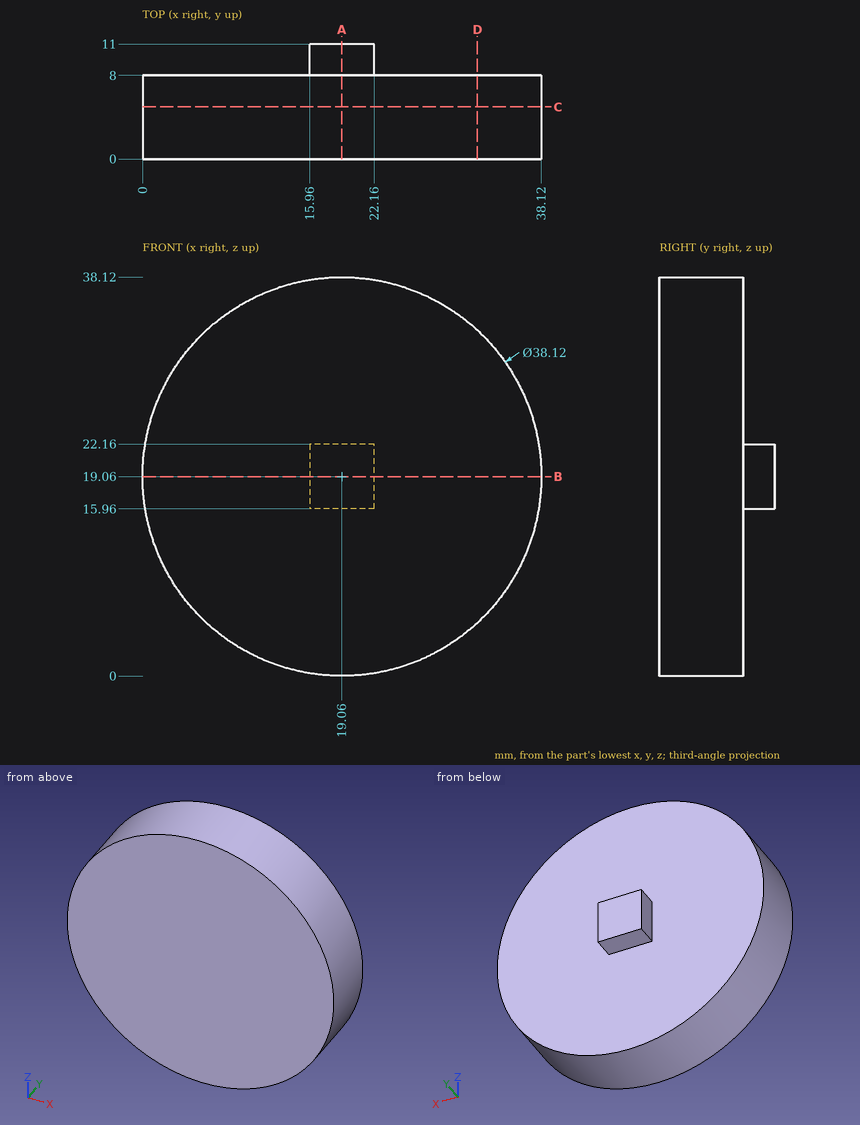
The figure shows three views and two pictorial views of one solid part (mm, origin at its lowest corner). Answer the questions. Round coordinates to 2 decimals unless told otherwise and drop trailing zeros. Order: outer loops, then holes, each group sorted by start corner. A loop starts at its lowest first (then second) coordinate and runs counter-clockwise, first axis right, second up. Notation, with made-up numbers: M -9.5,-18 L 40.5,-18 A18 ccw 40.5,13 Z; hole C 36,74.25 d9. An arc over 180 degrees is marked long. Put each result on its own line as item: value. Start each with the question number.
Q1. Section C-C, the plane y = 5 is taken. Write down the section's boundary in (x, z).
Q2. Straight lines are drawn through the part: L1, parallel to Y at x = 9, z = 33.5; L2, parallel to Z at x = 20, y = 10.25; L3, parallel to X at y = 5.75, z = 18.5. For each, find the intervals that lie inside material, in ascending order. Write a range as [from, to].
Q3. Flat-ended cylindrical pins translate along their axes: pin 1 (0.9 mm diameter, centred on x = 19, y = 9, fed in from -Z); pin 2 (1.5 mm diameter, centred on y = 10, z = 18, fed in from -X); pin 3 (2.5 mm diameter, centred on y = 9, z = 18, fed in from +X). Find the tip coordinate at first contact, or state that the pin passes through.
Q4. Section A-A, the plane x = 19.06 is taken. Write down the section's boundary in (y, z).
Q5. Section D-D, the plane x = 32 is taken. Write down the section's boundary in (y, z), and give its area (3 significant figures).
Q6. Section B-B, the plane z = 19.06 is taken. Write down the section's boundary in (x, y), and give its area (3 significant figures).
Findings below:
1. outline: C 19.06,19.06 d38.12
2. L1: y = [0, 8]
2. L2: z = [15.96, 22.16]
2. L3: x = [0.01, 38.11]
3. pin 1: stops at z = 15.96
3. pin 2: stops at x = 15.96
3. pin 3: stops at x = 38.12
4. outline: M 0,0 L 8,0 L 8,15.96 L 11,15.96 L 11,22.16 L 8,22.16 L 8,38.12 L 0,38.12 Z
5. outline: M 0,5.07 L 8,5.07 L 8,33.05 L 0,33.05 Z
5. area: 224 mm^2
6. outline: M 0,0 L 38.12,0 L 38.12,8 L 22.16,8 L 22.16,11 L 15.96,11 L 15.96,8 L 0,8 Z
6. area: 324 mm^2
